```python
from build123d import *

# Parameters (mm, degrees)
BOSS_EXTRUDE1_DEPTH = 1
SKETCH2_W           = 1
SKETCH2_H           = 1.8
SKETCH2_W_2         = 1.8
SKETCH2_H_2         = 1
BOSS_EXTRUDE2_DEPTH = 1


with BuildPart() as part:
    # Sketch1 → Boss-Extrude1 (new body)
    with BuildSketch(Plane(origin=(0, 0, 0), x_dir=(1, 0, 0), z_dir=(0, 1, 0))):
        Polygon((-25.606601718, 15), (-15, 25.606601718), (15, 25.606601718), (25.606601718, 15), (25.606601718, -15), (15, -25.606601718), (-15, -25.606601718), (-25.606601718, -15), align=None)
    extrude(amount=BOSS_EXTRUDE1_DEPTH)

    # Sketch2 → Boss-Extrude2 (add)
    with BuildSketch(Plane(origin=(0, 1, 0), x_dir=(1, 0, 0), z_dir=(0, 1, 0))):
        with Locations((-26.106601718, 0)):
            Rectangle(SKETCH2_W, SKETCH2_H)
        with Locations((0, 26.106601718)):
            Rectangle(SKETCH2_W_2, SKETCH2_H_2)
        with Locations((0, -26.106601718)):
            Rectangle(SKETCH2_W_2, SKETCH2_H_2)
        with Locations((26.106601718, 0)):
            Rectangle(SKETCH2_W, SKETCH2_H)
    extrude(amount=-BOSS_EXTRUDE2_DEPTH)


solid = part.part
```
Can you work these out from the model? Positions are in its coordinate system, mm. Round coordinates to 2 decimals unless told otherwise and drop trailing zeros. Loops run counter-clockwise (first coordinate to the right, second up) from the corner with the lowest first, then second, coordinate; pieces in that order, holes last. Notation, with made-up numbers: (-22.75, -2) -> (-17.75, -2) arc R20 cw to (-17.75, 13) -> close; hole circle Ø10 at (59.5, 56.5). An arc over 180 degrees is marked (long way). Answer in a Markdown table with one row per item.
Item 1: Suppose I cut it at B-B, the plane x = -10.5. List the corners of the cut face in (y, z) for me, plus the area to 3 significant figures.
Answer block:
| item | result |
|---|---|
| outline | (0, -25.61) -> (1, -25.61) -> (1, 25.61) -> (0, 25.61) -> close |
| area | 51.2 mm² |
Item 2: Will these pins go through, and if not, where does the flat tip stop? P1, Ø0.5, axis at x = 26, y = 0.5, coming from the +Z side; P2, Ø0.5, axis at y = 0.5, z = -26, coming from the -X side; P3, Ø0.5, axis at y = 0.5, z = 26.5, coming from the +X side.
Answer block:
| item | result |
|---|---|
| P1 | z = 0.9 |
| P2 | x = -0.9 |
| P3 | x = 0.9 |
Item 3: Suppose I cut it at A-A, the plane y = 0.15. List the corners of the cut face in (x, z) for me, plus the area to 3 significant figures.
Answer block:
| item | result |
|---|---|
| outline | (-26.61, -0.9) -> (-25.61, -0.9) -> (-25.61, -15) -> (-15, -25.61) -> (-0.9, -25.61) -> (-0.9, -26.61) -> (0.9, -26.61) -> (0.9, -25.61) -> (15, -25.61) -> (25.61, -15) -> (25.61, -0.9) -> (26.61, -0.9) -> (26.61, 0.9) -> (25.61, 0.9) -> (25.61, 15) -> (15, 25.61) -> (0.9, 25.61) -> (0.9, 26.61) -> (-0.9, 26.61) -> (-0.9, 25.61) -> (-15, 25.61) -> (-25.61, 15) -> (-25.61, 0.9) -> (-26.61, 0.9) -> close |
| area | 2,400 mm² |
Item 4: Suppose I cut it at C-C, the plane z = -3. List the corners of the cut face in (x, y) for me.
Answer block:
| item | result |
|---|---|
| outline | (-25.61, 0) -> (25.61, 0) -> (25.61, 1) -> (-25.61, 1) -> close |
Item 5: If I drill on probe 1 along X at (y, z) = (0.4, 14); probe 2 along X at (y, z) = (0.35, -24), over which ranges is the centre line in solid material (lowest first)?
Answer block:
| item | result |
|---|---|
| probe 1 | -25.61 to 25.61 |
| probe 2 | -16.61 to 16.61 |
